The drawing under review shows one solid part. Ordinate dimensions are in mm from its lowest x, y, z. A direction names the side the tool comes from. Coordinates: 2 decimals unless noted, no trailing zeros. Write each loop counter-clockwise with the first axis right and the second up, starting at its lowest first coordinate (ties: lowest second). Pieces come first, ordered by that corner, then holes. Notation, with made-up numbers: (66.5, 33.25) - (85.5, 33.25) arc R6 cw to (85.5, 42.25) - close; hole circle Ø1 at (73, 3.5). An arc over 180 degrees is marked (long way). Use a Markdown table: item, result.
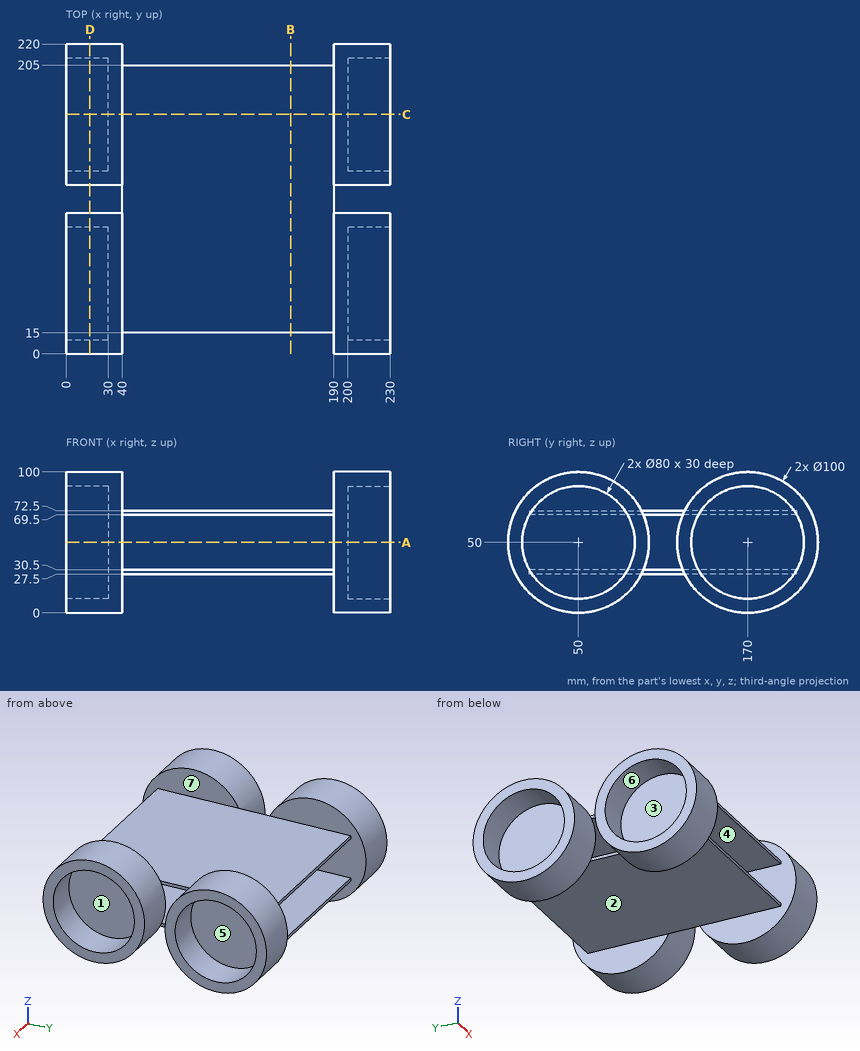
(1) Take a section at C-C on y = 170. Write out the cut boundary in (x, z), and give its area (3 significant figures).
Determined:
| item | result |
|---|---|
| outline | (0, 0) - (40, 0) - (40, 27.5) - (190, 27.5) - (190, 0) - (230, 0) - (230, 10) - (200, 10) - (200, 90) - (230, 90) - (230, 100) - (190, 100) - (190, 72.5) - (40, 72.5) - (40, 100) - (0, 100) - (0, 90) - (30, 90) - (30, 10) - (0, 10) - close; hole (40, 30.5) - (190, 30.5) - (190, 69.5) - (40, 69.5) - close |
| area | 4,100 mm2 |
(2) For L1, parallel to Y at x = 207, z = 48.5; L2, parallel to Z at x = 144.5, y = 193; L3, parallel to X at y = 16, z = 82, list the stretches that pass through material, from the lowest coordinate up. Write a range as from..to.
Determined:
| item | result |
|---|---|
| L1 | 0.02..10.03, 89.97..99.98, 120.02..130.03, 209.97..219.98 |
| L2 | 27.5..30.5, 69.5..72.5 |
| L3 | 0..40, 190..230 |
(3) Take a section at B-B on x = 159.5. Write out the cut boundary in (y, z), and give its area (3 significant figures).
Determined:
| item | result |
|---|---|
| outline | (15, 27.5) - (205, 27.5) - (205, 30.5) - (15, 30.5) - close; (15, 69.5) - (205, 69.5) - (205, 72.5) - (15, 72.5) - close |
| area | 1,140 mm2 |
(4) Draft analysis for pull direction X (two halves, no side actions). For the marked faces 5, 6 and 7, state which applies: +X half, -X half, draft (parallel to the pull), parting line (faces both ways), or undercut.
Determined:
| item | result |
|---|---|
| face 5 | +X half |
| face 6 | draft |
| face 7 | undercut |
(5) Take a section at A-A on z = 50. State how many separate pieces and enclosed holes the cut face has, and give its area (3 significant figures).
Determined:
| item | result |
|---|---|
| separate pieces | 4 |
| enclosed holes | 0 |
| area | 6,400 mm2 |
(6) For pin 1 (1.5 mm diameter, centred on x = 48, y = 136.5, fed in from -Z); pin 2 (2.5 mm diameter, centred on x = 111.5, z = 71, fed in from -Y); pin 3 (1.5 mm diameter, centred on x = 113, z = 28.5, fed in from +Y), all flat-tipped, find the tip position at first contact; note any pin that passes through.
Determined:
| item | result |
|---|---|
| pin 1 | z = 27.5 |
| pin 2 | y = 15 |
| pin 3 | y = 205 |
(7) Machinability: for the marked faces 1, 2, 3 and 4, which of the approach directions +Z, -Z, +X, -X, +Y, -Y give a long, thin tool a straight path to every point of the face, cutting with its end or side? Answer none if there is none.
Determined:
| item | result |
|---|---|
| face 1 | +X |
| face 2 | -Z, +Y, -Y |
| face 3 | -X |
| face 4 | +Y, -Y |
(8) Take a section at D-D on x = 17. Write out the cut boundary in (y, z), and give its area (3 significant figures).
Determined:
| item | result |
|---|---|
| outline | circle Ø100 at (50, 50); circle Ø100 at (170, 50); hole circle Ø80 at (50, 50); hole circle Ø80 at (170, 50) |
| area | 5,650 mm2 |
